Here's how the part is built. I have some questions about the finished solid (model axes, mm). Face numbers are marked on the shaded views. A direction names the side the tool comes from. Coordinates: 2 decimals unless noted, no trailing zeros. Write each loop counter-clockwise with the first axis right and the second up, starting at its lowest first coordinate (ties: lowest second). Pieces come first, ordered by that corner, then holes. Notation, with made-up numbers: (2.25, 83.5) -> (49.25, 83.5) arc R23 ccw to (49.25, 101.5) -> close; hole circle Ø10 at (15.5, 59.5). An arc over 180 degrees is marked (long way). Put each result on its own line as item: value. Start each with the question number.
Item 1: I need wall thicknesses on line 1 (Z direction, x = 0, y = 4.5); line 2 (X direction, y = 5.25, z = 0); line 3 (X direction, y = 8.5, z = 0). Which ranges of each line are inside material? Lowest first, please. Write a range as [from, to].
Item 2: On a 3-axis mill with a long thin cutter (end or side, diameter ignored), from which of +Z, -Z, +X, -X, +Y, -Y can I reach the whole of each face in a straight line? I mean the marked faces 5, 6, 7, 8 and 9. Say none if no direction works.
Item 3: I want a section at C-C, the plane x = 0. List the corners of the cut face in (y, z) for me, then the cut area to 3 significant figures.
Item 4: I want a section at D-D, the plane y = 7.75. List the corners of the cut face in (x, z) for me.
Item 5: I want a section at A-A, the plane y = 2.25. List the corners of the cut face in (x, z) for me (1 decimal), then the cut area to 3 significant figures.
Item 6: If we mould it in two halves opening along Z, with no side actions, what happens to the marked faces 1, 2, 3 and 4? For each: released by +Z, released by -Z, zero draft, split by the parting line, or undercut.
Item 7: For pin 1 (8 mm diameter, centred on x = 1.5, y = 14, fed in from -Z); pin 2 (3 mm diameter, centred on x = -20.5, y = 3, fed in from -Z); pin 3 (1 mm diameter, centred on y = 13, z = -6, fed in from +X), each with a flat end and sliding along its axis, tell me the tip position at first contact or that it passes through.
Item 8: I want a section at B-B, the plane z = 0. List the corners of the cut face in (x, y) for me, then the cut area to 3 significant figures.
from build123d import *

# Parameters (mm, degrees)
SKETCH1_R           = 33.3375
SKETCH1_R_2         = 21.5265
BOSS_EXTRUDE1_DEPTH = 6.35
SKETCH5_R           = 39.889033067
CUT_EXTRUDE2_DEPTH  = 6.35
SKETCH6_W           = 3.697979252
SKETCH6_H           = 3.723099818
CUT_EXTRUDE3_DEPTH  = 6.35


with BuildPart() as part:
    # Sketch1 → Boss-Extrude1 (new body)
    with BuildSketch(Plane(origin=(0, 0, 0), x_dir=(1, 0, 0), z_dir=(0, 1, 0))):
        with Locations(Location((0, 0, 0), (0, 0, 270))):
            Circle(SKETCH1_R)
        with Locations(Location((0, 0, 0), (0, 0, 270))):
            Circle(SKETCH1_R_2, mode=Mode.SUBTRACT)
    extrude(amount=BOSS_EXTRUDE1_DEPTH)

    # Sketch2 → Revolve1 (revolve)
    with BuildSketch(Plane.XY, mode=Mode.PRIVATE) as revolve1_sk:
        with BuildLine():
            Line((21.5265, 6.35), (21.5265, 17.82357951))
            ThreePointArc((21.5265, 17.82357951), (21.885975678, 18.30938248), (22.455651676, 18.107648632))
            Line((22.455651676, 18.107648632), (25.85475838, 13.068243159))
            ThreePointArc((25.85475838, 13.068243159), (26.17801485, 12.390519163), (26.289, 11.647897552))
            Line((26.289, 11.647897552), (26.289, 6.35))
            Line((26.289, 6.35), (21.5265, 6.35))
        make_face()
    revolve(revolve1_sk.sketch.rotate(Axis((0, 21.224675992, 0), (0, -1, 0)), 90), axis=Axis((0, 21.224675992, 0), (0, -1, 0)))

    # Sketch5 → Cut-Extrude2 (cut)
    with BuildSketch(Plane(origin=(0, 0, 0), x_dir=(1, 0, 0), z_dir=(0, 1, 0))):
        Circle(SKETCH5_R)
        with BuildLine():
            Line((-24.11485133, 23.01875), (-18.134546198, 23.01875))
            ThreePointArc((-18.134546198, 23.01875), (0, 29.304003436), (18.134546198, 23.01875))
            Line((18.134546198, 23.01875), (24.11485133, 23.01875))
            ThreePointArc((24.11485133, 23.01875), (28.871121899, 16.66875), (31.992247929, 9.374698861))
            Line((31.992247929, 9.374698861), (29.002095362, 4.195602693))
            ThreePointArc((29.002095362, 4.195602693), (25.378011408, -14.652001718), (10.867549165, -27.214352693))
            Line((10.867549165, -27.214352693), (7.877396598, -32.393448861))
            ThreePointArc((7.877396598, -32.393448861), (0, -33.3375), (-7.877396598, -32.393448861))
            Line((-7.877396598, -32.393448861), (-10.867549165, -27.214352693))
            ThreePointArc((-10.867549165, -27.214352693), (-25.378011408, -14.652001718), (-29.002095362, 4.195602693))
            Line((-29.002095362, 4.195602693), (-31.992247929, 9.374698861))
            ThreePointArc((-31.992247929, 9.374698861), (-28.871121899, 16.66875), (-24.11485133, 23.01875))
        make_face(mode=Mode.SUBTRACT)
    extrude(amount=CUT_EXTRUDE2_DEPTH, mode=Mode.SUBTRACT)

    # Sketch6 → Cut-Extrude3 (cut)
    with BuildSketch(Plane(origin=(0, 0, 0), x_dir=(1, 0, 0), z_dir=(0, 1, 0))):
        Polygon((-28.1834672, 14.136703058), (-31.407766223, 15.998252967), (-29.558776597, 19.200796942), (-26.334477574, 17.339247033), align=None)
        with Locations((0, -33.3375)):
            Rectangle(SKETCH6_W, SKETCH6_H)
        Polygon((26.334477574, 17.339247033), (29.558776597, 19.200796942), (31.407766223, 15.998252967), (28.1834672, 14.136703058), align=None)
    extrude(amount=CUT_EXTRUDE3_DEPTH, mode=Mode.SUBTRACT)


solid = part.part
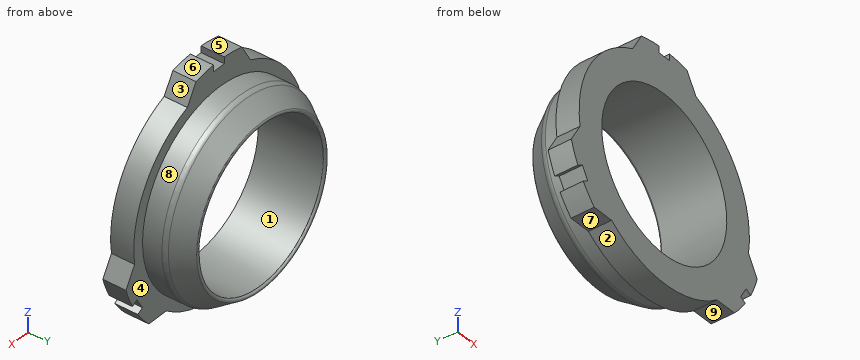
Calculated:
1. line 1: z = [-29.3, -21.53], [21.53, 31.48]
1. line 2: x = [-29.3, -21.53], [21.53, 29.3]
1. line 3: x = [-26.29, -21.53], [21.53, 26.29]
2. face 5: +Z, -X, +Y, -Y
2. face 6: +Z, +X, +Y, -Y
2. face 7: -Z, -X, +Y, -Y
2. face 8: +Y
2. face 9: -Z, +X, +Y, -Y
3. outline: (0, -29.3) -> (6.35, -29.3) -> (6.35, -26.29) -> (11.65, -26.29) arc R2.54 ccw to (13.07, -25.85) -> (18.11, -22.46) arc R0.51 ccw to (17.82, -21.53) -> (0, -21.53) -> close; (0, 21.53) -> (17.82, 21.53) arc R0.51 ccw to (18.11, 22.46) -> (13.07, 25.85) arc R2.54 ccw to (11.65, 26.29) -> (6.35, 26.29) -> (6.35, 31.48) -> (0, 31.48) -> close
3. area: 203 mm2
4. outline: circle Ø52.58 at (0, 0); hole circle Ø43.05 at (0, 0)
5. outline: (-32, -9.4) arc R33.3 ccw to (-29.8, -15) -> (-28.2, -14.1) -> (-26.3, -17.3) -> (-27.9, -18.2) arc R33.3 ccw to (-24.1, -23) -> (-18.1, -23) arc R29.3 ccw to (18.1, -23) -> (24.1, -23) arc R33.3 ccw to (27.9, -18.2) -> (26.3, -17.3) -> (28.2, -14.1) -> (29.8, -15) arc R33.3 ccw to (32, -9.4) -> (29, -4.2) arc R29.3 ccw to (10.9, 27.2) -> (7.9, 32.4) arc R33.3 ccw to (1.8, 33.3) -> (1.8, 31.5) -> (-1.8, 31.5) -> (-1.8, 33.3) arc R33.3 ccw to (-7.9, 32.4) -> (-10.9, 27.2) arc R29.3 ccw to (-29, -4.2) -> close; hole circle Ø43.1 at (0, 0)
5. area: 1,450 mm2
6. face 1: undercut
6. face 2: released by -Z
6. face 3: released by +Z
6. face 4: zero draft
7. pin 1: stops at z = -26.29
7. pin 2: stops at z = -23.02
7. pin 3: stops at x = 25.48
8. outline: (-29.3, 0) -> (-21.53, 0) -> (-21.53, 17.82) arc R0.51 ccw to (-22.46, 18.11) -> (-25.85, 13.07) arc R2.54 ccw to (-26.29, 11.65) -> (-26.29, 6.35) -> (-29.3, 6.35) -> close; (21.53, 0) -> (29.3, 0) -> (29.3, 6.35) -> (26.29, 6.35) -> (26.29, 11.65) arc R2.54 ccw to (25.85, 13.07) -> (22.46, 18.11) arc R0.51 ccw to (21.53, 17.82) -> close
8. area: 189 mm2
